Geometry: final body of the model. Coordinates: model frame, mm. Face numbers are marked on the shaded views. A direction names the side the tool comes from. Give positions to 0.01 mm unless a question says otherwise; leave off trailing zeros. Order: outer loops, then holes, each group sorted by start corner. A loop starts at its lowest first (then second) coordinate and runs counter-clockwise, first axis right, second up. Notation, with made-up numbers: (-39.5, -2.5) - (11.5, -2.5) arc R36 ccw to (11.5, 36.5) - close; hole circle Ø9 at (15.25, -40). An arc over 180 degrees is marked (long way). Write item = value, one per line. Start each with the question number.
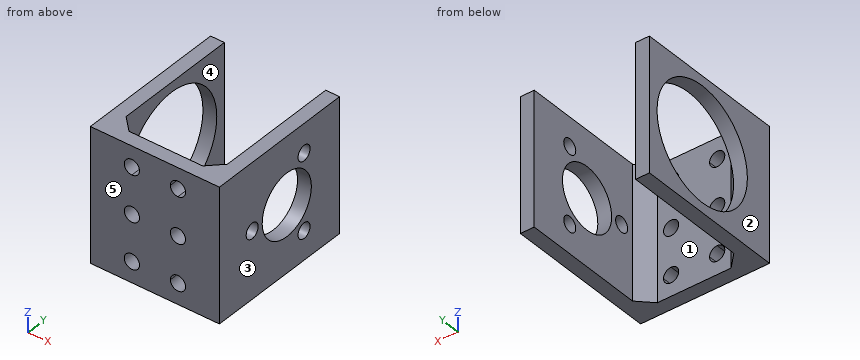
from build123d import *

# Parameters (mm, degrees)
SKETCH_1_W          = 28
SKETCH_1_H          = 29
EXTRUDE_1_DEPTH     = 3
SKETCH_2_W          = 3
SKETCH_2_H          = 29
EXTRUDE_2_DEPTH     = 30
SKETCH_3_R          = 1.65
CUT_EXTRUDE_1_DEPTH = 33
EXTRUDE_3_DEPTH     = 29
SKETCH_6_R          = 12.4
CUT_EXTRUDE_2_DEPTH = 5
SKETCH_8_R          = 1.65
CUT_EXTRUDE_3_DEPTH = 5
SKETCH_9_R          = 6.75
CUT_EXTRUDE_4_DEPTH = 5


with BuildPart() as part:
    # 草图1 → 凸台-拉伸1 (new body)
    with BuildSketch(Plane(origin=(0, 0, 0), x_dir=(1, 0, 0), z_dir=(0, 1, 0))):
        Rectangle(SKETCH_1_W, SKETCH_1_H)
    extrude(amount=EXTRUDE_1_DEPTH)

    # 草图2 → 凸台-拉伸2 (add)
    with BuildSketch(Plane(origin=(0, 3, 0), x_dir=(1, 0, 0), z_dir=(0, 1, 0))):
        with Locations((12.5, 0)):
            Rectangle(SKETCH_2_W, SKETCH_2_H)
        with Locations((-12.5, 0)):
            Rectangle(SKETCH_2_W, SKETCH_2_H)
    extrude(amount=EXTRUDE_2_DEPTH)

    # 草图3 → 切除-拉伸1 (cut)
    with BuildSketch(Plane.ZY.offset(14)):
        with Locations((-8.227241336, 23.25)):
            Circle(SKETCH_3_R)
        with Locations((8.227241336, 23.25)):
            Circle(SKETCH_3_R)
        with Locations((0, 9)):
            Circle(SKETCH_3_R)
    extrude(amount=-CUT_EXTRUDE_1_DEPTH, mode=Mode.SUBTRACT)

    # 草图5 → 凸台-拉伸3 (add)
    with BuildSketch(Plane(origin=(0, 0, -14.5), x_dir=(-1, 0, 0), z_dir=(0, 0, -1))):
        Polygon((11, 3), (11, 6), (8, 3), align=None)
        Polygon((-11, 3), (-11, 6), (-8, 3), align=None)
    extrude(amount=-EXTRUDE_3_DEPTH)

    # 草图6 → 切除-拉伸2 (cut)
    with BuildSketch(Plane.ZY.offset(14)):
        with Locations((0, 18.5)):
            Circle(SKETCH_6_R)
    extrude(amount=-CUT_EXTRUDE_2_DEPTH, mode=Mode.SUBTRACT)

    # 草图8 → 切除-拉伸3 (cut)
    with BuildSketch(Plane(origin=(0, 3, 0), x_dir=(1, 0, 0), z_dir=(0, 1, 0))):
        with BuildLine():
            ThreePointArc((-3.35, 10), (-6.166726189, 11.166726189), (-5, 8.35))
            Line((-5, 8.35), (-5, 10))
            Line((-5, 10), (-3.35, 10))
        make_face()
        with BuildLine():
            Line((-5, 10), (-5, 8.35))
            ThreePointArc((-5, 8.35), (-3.833273811, 8.833273811), (-3.35, 10))
            Line((-3.35, 10), (-5, 10))
        make_face()
        with BuildLine():
            ThreePointArc((3.35, 10), (3.833273811, 8.833273811), (5, 8.35))
            Line((5, 8.35), (5, 10))
            Line((5, 10), (3.35, 10))
        make_face()
        with BuildLine():
            Line((5, 10), (5, 8.35))
            ThreePointArc((5, 8.35), (6.166726189, 8.833273811), (6.65, 10))
            ThreePointArc((6.65, 10), (5, 11.65), (3.35, 10))
            Line((3.35, 10), (5, 10))
        make_face()
        with BuildLine():
            ThreePointArc((5, -8.35), (3.833273811, -8.833273811), (3.35, -10))
            Line((3.35, -10), (5, -10))
            Line((5, -10), (5, -8.35))
        make_face()
        with BuildLine():
            Line((5, -10), (3.35, -10))
            ThreePointArc((3.35, -10), (5, -11.65), (6.65, -10))
            ThreePointArc((6.65, -10), (6.166726189, -8.833273811), (5, -8.35))
            Line((5, -8.35), (5, -10))
        make_face()
        with BuildLine():
            Line((-5, -8.35), (-5, -10))
            Line((-5, -10), (-3.35, -10))
            ThreePointArc((-3.35, -10), (-3.833273811, -8.833273811), (-5, -8.35))
        make_face()
        with BuildLine():
            Line((-3.35, -10), (-5, -10))
            Line((-5, -10), (-5, -8.35))
            ThreePointArc((-5, -8.35), (-6.166726189, -11.166726189), (-3.35, -10))
        make_face()
        with Locations(Location((5, 0, 0), (0, 0, 270))):
            Circle(SKETCH_8_R)
        with Locations(Location((-5, 0, 0), (0, 0, 270))):
            Circle(SKETCH_8_R)
    extrude(amount=-CUT_EXTRUDE_3_DEPTH, mode=Mode.SUBTRACT)

    # 草图9 → 切除-拉伸4 (cut)
    with BuildSketch(Plane(origin=(14, 0, 0), x_dir=(0, 0, -1), z_dir=(1, 0, 0))):
        with Locations((0, 18.5)):
            Circle(SKETCH_9_R)
    extrude(amount=-CUT_EXTRUDE_4_DEPTH, mode=Mode.SUBTRACT)


solid = part.part
Q1. Pull-direction query (X, two-part tool) for the marked faces 1, 2 and 3; classes: +X half, -X half, draft (parallel to the pull), parting line (faces both ways), or undercut.
Q2. Material intervals for line 1 along Y through (x, z) = (11.9, 0); line 2 along X through (y, z) = (0.85, -10); line 3 along X through (y, z) = (32.5, -9.5), sorted ascending. Write a range as from..to.
Q3. Section A-A, the plane x = 11.75. Return the cut outline in (y, z), then the cut area to 3 significant figures.
Q4. Section C-C, the plane y = 4. Return the cut outline in (x, z).
Q5. Section D-D, the plane y = 23.25. Return the cut outline in (x, z), then the cut area to 3 significant figures.
Q6. Set-up query: the marked faces 4 and 5. Return all of +Z, -Z, +X, -X, +Y, -Y with unobstructed straight access to the full face (end or side cutting, diameter ignored); none if empty.
Q7. Contact query for flat-ended pins moving along their axis: pin 1 (2 mm diameter, centred on x = -3.5, z = -10, fed in from +Y); pin 2 (13.5 mm diameter, centred on y = 23, z = 2, fed in from -X); pin 3 (10 mm diameter, centred on x = -5.5, z = 2.5, fed in from +Y). Output: stop coordinate, or through.
Q8. Section B-B, the plane z = 0. Count the separate pieces of the cut face and the enclosed holes in it, then the cut area to 3 significant figures.
The answers:
q1.face_1 = undercut
q1.face_2 = -X half
q1.face_3 = +X half
q2.line_1 = 0..7.35, 10.65..11.75, 25.25..33
q2.line_2 = -14..-6.65, -3.35..3.35, 6.65..14
q2.line_3 = -14..-11, 11..14
q3.outline = (0, -14.5) - (33, -14.5) - (33, 14.5) - (0, 14.5) - close; hole circle Ø3.3 at (9, 0); hole circle Ø13.5 at (18.5, 0); hole circle Ø3.3 at (23.25, -8.23); hole circle Ø3.3 at (23.25, 8.23)
q3.area = 788 mm²
q4.outline = (-14, -14.5) - (-9, -14.5) - (-9, 14.5) - (-14, 14.5) - close; (9, -14.5) - (14, -14.5) - (14, 14.5) - (9, 14.5) - close
q5.outline = (-14, -14.5) - (-11, -14.5) - (-11, -11.45) - (-14, -11.45) - close; (-14, 11.45) - (-11, 11.45) - (-11, 14.5) - (-14, 14.5) - close; (11, -14.5) - (14, -14.5) - (14, -9.88) - (11, -9.88) - close; (11, -6.58) - (14, -6.58) - (14, -4.8) - (11, -4.8) - close; (11, 4.8) - (14, 4.8) - (14, 6.58) - (11, 6.58) - close; (11, 9.88) - (14, 9.88) - (14, 14.5) - (11, 14.5) - close
q5.area = 56.7 mm²
q6.face_4 = +Z, -Z, +Y
q6.face_5 = +Z, -Z, +X, -X, -Y
q7.pin_1 = 3
q7.pin_2 = 11
q7.pin_3 = 5.5
q8.separate_pieces = 6
q8.enclosed_holes = 0
q8.area = 128 mm²
